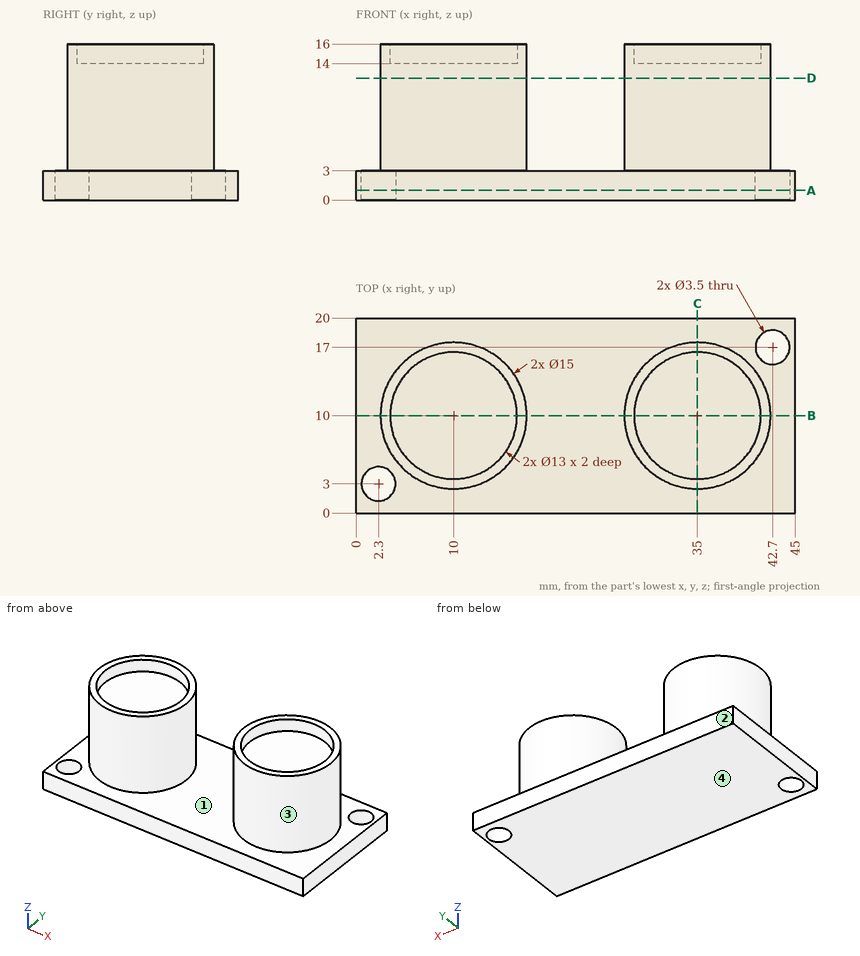
The figure shows three views and two pictorial views of one solid part (mm, origin at its lowest corner). Answer the questions. A direction names the side the tool comes from. Coordinates: 2 decimals unless noted, no trailing zeros. Loops run counter-clockwise (first coordinate to the right, second up) from the corner with the lowest first, then second, coordinate; pieces in that order, holes last. Notation, with made-up numbers: M -22,-22.75 L 21,-22.75 A13 ccw 21,-18.75 Z; hole C 15,19 d8. An arc over 180 degrees is marked long. Use CSV: the item, a comma, the result in double quotes. Start each with the question number.
(1) For a pull along X with two mould halves and no side action, classify the marked faces 3 and 4 as +X half, -X half, draft (parallel to the pull), parting line (faces both ways), or undercut.
(2) Find section C-C, the plane x = 35. Give the vertices of the cut face in (y, z), then the cut area to 3 significant figures.
(3) Find section B-B, the plane y = 10. Give the vertices of the cut face in (x, z), then the cut area to 3 significant figures.
(4) Consider line 1 (Y direction, x = 10, z = 15.05); line 2 (Y direction, x = 42.7, z = 1.4); line 3 (Z direction, x = 40.5, y = 8.75). Determine where each line is inside the solid, lowest interval first.
(5) Find section D-D, the plane z = 12.5. Give the vertices of the cut face in (x, y).
(6) For the marked faces 1 and 2, determine the directions among +Z, -Z, +X, -X, +Y, -Y from which every point of the face is accessible in a straight line to the end or side of a thin tool.
(7) Find section A-A, the plane z = 1. Give the vertices of the cut face in (x, y).
(8) Given pin 1 Ø3 at (x, z) = (27.5, 9) entering from -Y; pin 2 Ø6.5 at (x, y) = (33, 10.5) entering from +Z; pin 3 Ø2 at (x, y) = (42.7, 17) entering from -Z; pin 4 Ø8 at (y, z) = (12, 14.5) entering from +X, each flat-ended and moving along its own axis, determine where each tip first touches the part or whether it passes through.
Recorded:
1,face 3,"undercut"
1,face 4,"draft"
2,outline,"M 0,0 L 20,0 L 20,3 L 17.5,3 L 17.5,16 L 16.5,16 L 16.5,14 L 3.5,14 L 3.5,16 L 2.5,16 L 2.5,3 L 0,3 Z"
2,area,"229 mm^2"
3,outline,"M 0,0 L 45,0 L 45,3 L 42.5,3 L 42.5,16 L 41.5,16 L 41.5,14 L 28.5,14 L 28.5,16 L 27.5,16 L 27.5,3 L 17.5,3 L 17.5,16 L 16.5,16 L 16.5,14 L 3.5,14 L 3.5,16 L 2.5,16 L 2.5,3 L 0,3 Z"
3,area,"473 mm^2"
4,line 1,"y = 2.5 to 3.5, 16.5 to 17.5"
4,line 2,"y = 0 to 15.25, 18.75 to 20"
4,line 3,"z = 0 to 14"
5,outline,"C 10,10 d15; C 35,10 d15"
6,face 1,"+Z"
6,face 2,"+Z, -Z, +X, -X, +Y"
7,outline,"M 0,0 L 45,0 L 45,20 L 0,20 Z; hole C 2.3,3 d3.5; hole C 42.7,17 d3.5"
8,pin 1,"stops at y = 5.5"
8,pin 2,"stops at z = 14"
8,pin 3,"passes through"
8,pin 4,"stops at x = 42.5"
